Check sheet for the modelled part. Datum: model origin and axes. Units: mm. Coordinates: 2 decimals unless noted, no trailing zeros. Loops run counter-clockwise (first coordinate to the right, second up) from the corner with the lowest first, then second, coordinate; pieces in that order, holes last.
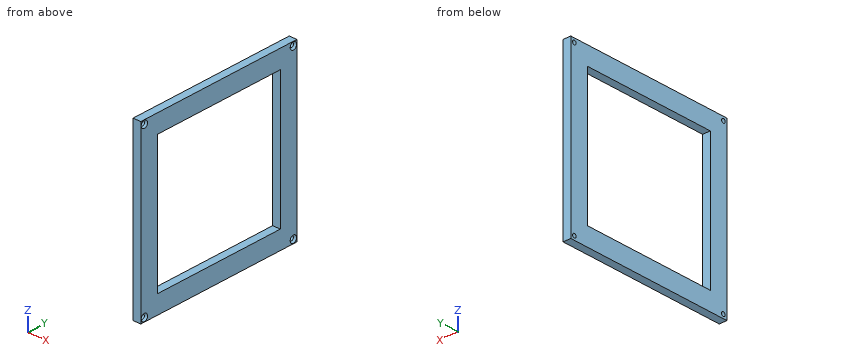
Autodesk Inventor part; units mm, degrees
ref_plane "YZ Plane" through (0, 0, 0) normal (1, 0, 0) x (0, 1, 0)
ref_plane "XZ Plane" through (0, 0, 0) normal (0, 1, 0) x (-1, 0, 0)
ref_plane "XY Plane" through (0, 0, 0) normal (0, 0, 1) x (1, 0, 0)
sketch "Sketch1" plane through (0, 0, 0) normal (1, 0, 0) x (0, 1, 0)
  line L0 (-69.85, -69.85) -> (69.85, -69.85)
  line L1 (69.85, -69.85) -> (69.85, 69.85)
  line L2 (69.85, 69.85) -> (-69.85, 69.85)
  line L3 (-69.85, 69.85) -> (-69.85, -69.85)
  line L4 (-69.85, -69.85) -> (69.85, 69.85) construction
  line L5 (69.85, -69.85) -> (-69.85, 69.85) construction
  point P0 (0, 0)
  dimension "d0" = 139.7
  dimension "d1" = 139.7
extrude "Extrusion1" add sketch "Sketch1" along normal blind 6.35
sketch "Sketch26" plane through (6.35, 0, 0) normal (1, 0, 0) x (0, 0, -1)
  line L0 (69.85, -69.85) -> (69.85, 69.85)
  line L1 (69.85, 69.85) -> (-69.85, 69.85)
  line L2 (-69.85, 69.85) -> (-69.85, -69.85)
  line L3 (-69.85, -69.85) -> (69.85, -69.85)
  point P0 (0, 0)
  point P1 (-66.675, -66.675)
  dimension "d247" = 3.175
  dimension "d248" = 3.175
hole "Hole14" at (6.35, -66.675, 66.675) direction (-1, 0, 0) diameter 3.264 end through all countersink diameter 5.715 countersink angle 82
pattern_circular "Circular Pattern1" count 4 over 360 about axis through (-10, 0, 0) along (1, 0, 0) of "Hole14"
sketch "Sketch27" plane through (6.35, 0, 0) normal (1, 0, 0) x (0, 0, -1)
  circle A0 centre (-66.675, 66.675) radius 2.8575
  circle A1 centre (66.675, 66.675) radius 2.8575
  circle A2 centre (66.675, -66.675) radius 2.8575
  circle A3 centre (-66.675, -66.675) radius 2.8575
  line L0 (69.85, -69.85) -> (69.85, 69.85)
  line L1 (69.85, 69.85) -> (-69.85, 69.85)
  line L2 (-69.85, 69.85) -> (-69.85, -69.85)
  line L3 (-69.85, -69.85) -> (69.85, -69.85)
  line L4 (55, -55) -> (-55, -55)
  line L5 (-55, -55) -> (-55, 55)
  line L6 (-55, 55) -> (55, 55)
  line L7 (55, 55) -> (55, -55)
  line L8 (55, -55) -> (-55, 55) construction
  line L9 (-55, -55) -> (55, 55) construction
  point P0 (0, 0)
  dimension "d259" = 110
  dimension "d260" = 110
extrude "Extrusion12" cut sketch "Sketch27" against normal through all contours L4 L5 L6 L7
equation "\"height\" = 127"
equation "\"frameAcrylicThickness\" = 9.525"
equation "\"internalAcrylicThickness\" = 6.35"
equation "\"width\" = 127"
equation "\"depth\" = 146.05"
equation "\"mirrorAngle\" = 5deg"
equation "\"detectorWidth\" = 52"
equation "\"detectorHeight\" = 52"
equation "\"mirrorThickness\" = 3.175"
equation "\"fresnelThickness\" = 0.1"
equation "\"focalLength\" = 76.2"
equation "\"ior\" = 1.49"
equation "\"centerThickness\" = 1.524"
equation "\"fresnelAngle\" = 90deg"
equation "\"fresnelEffectiveDiameter\" = 152.4"
equation "\"oRingWidth\" = 1.5875"
equation "\"sensorHolderDepth\" = 19.05"
equation "\"aerogelClearence\" = 3.175"
equation "\"backplanePCBHeight\" = 76.2"
equation "\"backplanePCBWidth\" = 76.2"
equation "\"backplaneHoleOffsett\" = 6.35"
equation "\"backplanePostionOffsett\" = 12.7"
equation "\"moduleSlotClearence\" = 0.79375"
equation "\"plasticThickness\" = 6.35"
equation "\"aerogelHolderDepth\" = 37.30625"
properties part number "back" material "PC/ABS Plastic"
1) Section check A-A on z = -17. Enter the section's corners in (x, y).
Answer sheet:
outline: (0, -69.85) - (6.35, -69.85) - (6.35, -55) - (0, -55) - close; (0, 55) - (6.35, 55) - (6.35, 69.85) - (0, 69.85) - close
2) Depth check by flat-ended pin: pin 1 (5 mm diameter, centred on y = 66.675, z = -66.675, fed in from +X); pin 2 (4 mm diameter, centred on y = -66.675, z = -66.675, fed in from +X). Enter the tip coordinate at first touch or a pass-through.
Answer sheet:
pin 1: stops at x = 5.94
pin 2: stops at x = 5.36
3) Scan line: line 1 (Z direction, x = 5.5, y = 39). Record every from-to range of solid material in increasing order.
Answer sheet:
line 1: z = -69.85 to -55, 55 to 69.85
4) Section check C-C on x = 2.75. Enter the section's corners in (y, z) (3 decimals).
Answer sheet:
outline: (-69.85, -69.85) - (69.85, -69.85) - (69.85, 69.85) - (-69.85, 69.85) - close; hole circle Ø3.264 at (-66.675, -66.675); hole circle Ø3.264 at (-66.675, 66.675); hole (-55, -55) - (55, -55) - (55, 55) - (-55, 55) - close; hole circle Ø3.264 at (66.675, -66.675); hole circle Ø3.264 at (66.675, 66.675)
